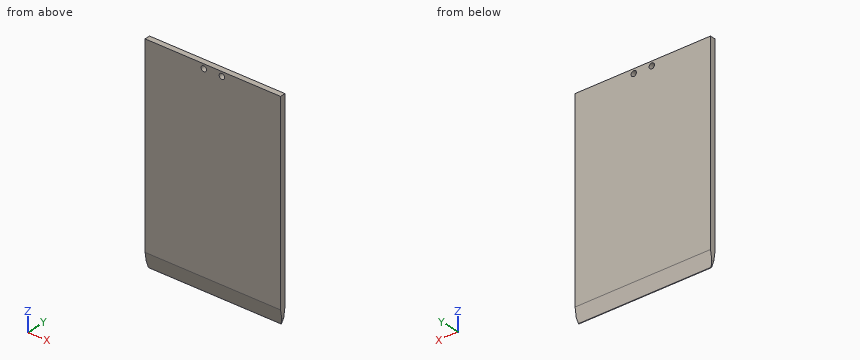
```python
from build123d import *

# Parameters (mm, degrees)
F1_DEPTH = 225
F2_R     = 9
F3_DEPTH = 25


with BuildPart() as f1:
    # F0 (on Right) → F1 (new body, symmetric)
    with BuildSketch(Plane.YZ):
        with BuildLine():
            Line((9, -299.5), (9, 348.5))
            Line((9, 348.5), (-9, 348.5))
            Line((-9, 348.5), (-9, -299.5))
            Line((-9, -299.5), (-0.98644, -347.664124))
            ThreePointArc((-0.98644, -347.664124), (-0.082342, -346.503396), (1, -347.5))
            ThreePointArc((1, -347.5), (0.996604, -347.582342), (0.98644, -347.664124))
            Line((0.98644, -347.664124), (9, -299.5))
        make_face()
        with BuildLine():
            ThreePointArc((0, -348.5), (0.646481, -348.26293), (0.98644, -347.664124))
            ThreePointArc((0.98644, -347.664124), (0.996604, -347.582342), (1, -347.5))
            ThreePointArc((1, -347.5), (-0.082342, -346.503396), (-0.98644, -347.664124))
            ThreePointArc((-0.98644, -347.664124), (-0.646481, -348.26293), (0, -348.5))
        make_face()
    extrude(amount=F1_DEPTH, both=True)

    # F2 (on face) → F3 (cut)
    with BuildSketch(Plane(origin=(0, 9, 0), x_dir=(-1, 0, 0), z_dir=(0, 1, 0))):
        with Locations((30, 333.5)):
            Circle(F2_R)
        with BuildLine():
            ThreePointArc((-39, 333.5), (-30, 324.5), (-21, 333.5))
            ThreePointArc((-21, 333.5), (-30, 342.5), (-39, 333.5))
        make_face()
        Polygon((-220.070133, -348.5), (-225, -329.500129), (-225.070133, -348.5), align=None)
        Polygon((225.070133, -348.5), (225, -329.500129), (220.070133, -348.5), align=None)
    extrude(amount=-F3_DEPTH, mode=Mode.SUBTRACT)


solid = f1.part
```
Can you work these out from the model? Positions are in its coordinate system, mm. Give positions to 0.01 mm unless a question says otherwise; leave off trailing zeros. Loops run counter-clockwise (first coordinate to the right, second up) from the corner with the lowest first, then second, coordinate; pieces in that order, holes last. Notation, with made-up numbers: M 87.5,55 L 113.5,55 A22 cw 113.5,94 Z; hole C -12,-3.75 d2. An arc over 180 degrees is marked long. Answer in a Markdown table with one row per item.
1. For pin 1 Ø4 at (x, y) = (-129.5, 1) entering from -Z, with a flat end and sliding along its axis, tell me the tip position at first contact or that it passes through.
Taken from the geometry:
| item | result |
|---|---|
| pin 1 | stops at z = -348.5 |
2. Suppose I cut it at B-B on z = 333.5. Write out the boundary of the cut face in (x, y).
Taken from the geometry:
| item | result |
|---|---|
| outline | M -225,-9 L -39,-9 L -39,9 L -225,9 Z; M -21,-9 L 21,-9 L 21,9 L -21,9 Z; M 39,-9 L 225,-9 L 225,9 L 39,9 Z |
3. Suppose I cut it at C-C on x = -46.5. Write out the boundary of the cut face in (y, z), plus the area to 3 significant figures.
Taken from the geometry:
| item | result |
|---|---|
| outline | M -9,-299.5 L -0.99,-347.66 A1 ccw 0.99,-347.66 L 9,-299.5 L 9,348.5 L -9,348.5 Z |
| area | 12,100 mm² |
4. If I drill on line 1 along Z through (x, y) = (-30, -0.5); line 2 along Z through (x, y) = (30, 0); line 3 along Y through (x, z) = (-171, -316), over which ranges is the centre line in solid material (lowest first)?
Taken from the geometry:
| item | result |
|---|---|
| line 1 | z = -348.37 to 324.5, 342.5 to 348.5 |
| line 2 | z = -348.5 to 324.5, 342.5 to 348.5 |
| line 3 | y = -6.25 to 6.25 |
5. Suppose I cut it at A-A on x = 30. Write out the boundary of the cut face in (y, z).
Taken from the geometry:
| item | result |
|---|---|
| outline | M -9,-299.5 L -0.99,-347.66 A1 ccw 0.99,-347.66 L 9,-299.5 L 9,324.5 L -9,324.5 Z; M -9,342.5 L 9,342.5 L 9,348.5 L -9,348.5 Z |
